Here's how the part is built. I have some questions about the finished solid (model axes, mm). A direction names the side the tool comes from. Round coordinates to 2 decimals unless told otherwise and drop trailing zeros. Loops run counter-clockwise (first coordinate to the right, second up) from the corner with the lowest first, then second, coordinate; pieces in that order, holes last. Notation, with made-up numbers: M 12,-30 L 32,-30 A30 cw 32,-7 Z; hole C 54.25,-12.5 d3. An arc over 180 degrees is marked long. Write each question's results on one line, items separated by ' | '. Start each with the question number.
Autodesk Fusion 360 part; units mm, degrees
sketch "Sketch1" plane through (0, 0, 0) normal (0, 0, 1) x (1, 0, 0)
  line L0 (3, 6) -> (38, 6)
  line L1 (38, 6) -> (38, -1)
  line L2 (38, -1) -> (3, -1)
  line L3 (3, -1) -> (3, 6)
  line L4 (3, 6) -> (5, 6)
  line L5 (5, 6) -> (5, -1)
  line L6 (5, -1) -> (3, -1)
  line L7 (3, -1) -> (3, 6)
  line L8 (5, 2.5) -> (12, 2.5)
  line L9 (12, 2.5) -> (12, 4)
  line L10 (12, 4) -> (5, 4)
  line L11 (5, 4) -> (5, 2.5)
  line L12 (5, 2.5) -> (12, 2.5)
  line L13 (12, 2.5) -> (12, 1)
  line L14 (12, 1) -> (5, 1)
  line L15 (5, 1) -> (5, 2.5)
  circle A0 centre (6.5, 2.5) radius 1.5
  circle A1 centre (10.5, 2.5) radius 1.5
  line L16 (3, -1) -> (13, -1)
  line L17 (13, -1) -> (13, 6)
  line L18 (13, 6) -> (3, 6)
  line L19 (3, 6) -> (3, -1)
  line L20 (13, 2.5) -> (20, 2.5)
  line L21 (20, 2.5) -> (20, 16)
  line L22 (20, 16) -> (13, 16)
  line L23 (13, 16) -> (13, 2.5)
  line L24 (13, 2.5) -> (20, 2.5)
  line L25 (20, 2.5) -> (20, -11)
  line L26 (20, -11) -> (13, -11)
  line L27 (13, -11) -> (13, 2.5)
  line L28 (20, 16) -> (20, 14)
  line L29 (13, 14) -> (13, 16)
  line L30 (13, -11) -> (20, -11)
  line L31 (20, -11) -> (20, -9)
  line L32 (13, -9) -> (13, -11)
  line L33 (20, -11) -> (20, -4)
  line L34 (20, -4) -> (13, -4)
  line L35 (13, -4) -> (13, -11)
  circle A2 centre (16.5, -7.5) radius 3.5
  circle A3 centre (16.5, -7.5) radius 1.5
  line L36 (13, 16) -> (20, 16)
  line L37 (20, 16) -> (20, 9)
  line L38 (20, 9) -> (13, 9)
  line L39 (13, 9) -> (13, 16)
  circle A4 centre (16.5, 12.5) radius 3.5
  circle A5 centre (16.5, 12.5) radius 1.5
  line L40 (38, 2.5) -> (23, 2.5)
  line L41 (23, 2.5) -> (23, 10)
  line L42 (23, 10) -> (38, 10)
  line L43 (38, 10) -> (38, 2.5)
  line L44 (23, 2.5) -> (38, 2.5)
  line L45 (38, 2.5) -> (38, -5)
  line L46 (38, -5) -> (23, -5)
  line L47 (23, -5) -> (23, 2.5)
  circle A6 centre (30.5, 2.5) radius 7.5
  circle A7 centre (30.5, 2.5) radius 1.5
  circle A8 centre (22.5, -3.5) radius 2.5
  circle A9 centre (22.5, 8.5) radius 2.5
  circle A10 centre (6.5, 2.5) radius 3.5
  circle A11 centre (10.5, 8.5) radius 2.5
  circle A12 centre (10.5, -3.5) radius 2.5
  dimension "d1" = 35
  dimension "d2" = 7
  dimension "d3" = 2
  dimension "d4" = 7
  dimension "d5" = 1.5
  dimension "d6" = 3
  dimension "d7" = 3
  dimension "d10" = 10
  dimension "d11" = 7
  dimension "d12" = 13.5
  dimension "d13" = 13.5
  dimension "d17" = 7
  dimension "d18" = 3
  dimension "d19" = 7
  dimension "d20" = 3
  dimension "d21" = 15
  dimension "d22" = 7.5
  dimension "d23" = 7.5
  dimension "d24" = 15
  dimension "d25" = 3
  dimension "d26" = 5
  dimension "d27" = 5
  dimension "d30" = 7
  dimension "d31" = 5
  dimension "d32" = 5
extrude "Extrude1" add sketch "Sketch1" along normal blind 2 contours L0 L3 L4 L5 L7 L18 L19 A10 | L0 L5 L18 A10 | L2 L3 L5 L6 L7 L16 L19 A10 | L5 L11 L15 A10 | L0 L2 L9 L10 L13 L14 L16 L17 L18 L23 L27 A10 | L5 L10 A10 | L2 L5 L16 A10 | L5 L14 A10 | L5 L10 L11 A0 | L5 L14 L15 A0 | L0 L21 L23 L38 | L0 L17 L20 L21 L23 L24 | L9 L10 A1 | L0 L21 A9 | L0 L2 L21 L25 L41 L47 | L2 L17 L20 L24 L25 L27 | L23 L38 L39 A4 | L13 L14 A1 | L2 L25 L27 L34 | A4 | L21 L37 L38 A4 | L2 L25 A8 | L27 L34 L35 A2 | L0 L41 A6 | A2 | L25 L33 L34 A2 | L0 A6 | L0 L40 L44 A6 A7 | L2 L47 A6 | L2 L40 L44 A6 A7 | L2 A6
extrude "Extrude2" add sketch "Sketch1" along normal blind 2 contours L2 L16 L27 A12
extrude "Extrude3" add sketch "Sketch1" along normal blind 2 contours L0 L18 L23 A11
extrude "Extrude4" cut sketch "Sketch1" along normal blind 2 contours L0 L3 L4 L5 L7 L18 L19 A10
extrude "Extrude5" cut sketch "Sketch1" along normal blind 2 contours L0 L5 L18 A10 | L2 L3 L5 L6 L7 L16 L19 A10 | L2 L5 L16 A10
Item 1: If we mould it in two halves opening along Y, with no side actions, what happens to faces 4 (the face through (9, 4, 1)), 5 (the face through (37.995, 2.779, 0.986)), 6 (the face through (20, 10, 1)), 7 (the face through (15, 12.43, 0.99))? For each: released by +Y, released by -Y, zero draft, split by the parting line, or undercut.
Item 2: If we section it at C-C on y = -1.75: Please give me the cut outline in (x, z).
Item 3: If we section it at A-A on x = 16.5: Please give me the cut outline in (y, z), and give its area (3 significant figures).
Item 4: I need wall thicknesses on L1, parallel to Y at x = 16.5, z = 0.55; L2, parallel to X at y = 2.5, z = 1.1; L3, parallel to X at y = 3.75, z = 0.45. Which ranges of each line are inside material? Lowest first, please.
Item 5: If we section it at B-B on z = 1.5: Please give me the cut outline in (x, y), and give its area (3 significant figures).
Item 6: Which directions (+Z, -Z, +X, -X, +Y, -Y) give clear straight access to the entire face, cutting with the end or side of a thin tool? Please do faces 1 (the face through (13, 11, 1)), 2 (the face through (20, -5, 1)), 3 (the face through (20.752, 6.713, 0.986)).
Item 7: If we section it at D-D on x = 8: Please give me the cut outline in (y, z), and give its area (3 significant figures).
Item 8: I'm going to push flat-ended pins straight in: pin 1 (0.6 mm diameter, centred on x = 8, z = 1.5, fed in from -Y); pin 2 (1.8 mm diameter, centred on x = 30.5, y = 2.5, fed in from -Z); pin 3 (0.6 mm diameter, centred on y = -6, z = 0.5, fed in from -X). Where does each tip first touch, or does it pass through?
Numbers:
1) face 4: undercut | face 5: split by the parting line | face 6: zero draft | face 7: undercut
2) outline: M 12.29,0 L 20.71,0 L 20.71,2 L 12.29,2 Z; M 24.32,0 L 36.68,0 L 36.68,2 L 24.32,2 Z
3) outline: M -11,0 L -9,0 L -9,2 L -11,2 Z; M -6,0 L 11,0 L 11,2 L -6,2 Z; M 14,0 L 16,0 L 16,2 L 14,2 Z | area: 42.0 mm²
4) L1: -11 to -9, -6 to 11, 14 to 16 | L2: 3 to 5, 12 to 29, 32 to 38 | L3: 3.23 to 5.67, 11.33 to 29.67, 31.33 to 37.9
5) outline: M 6.5,-1 L 10.5,-1 A2.5 cw 13,-3.5 L 13,-7.5 A3.5 ccw 20,-7.5 L 20,-3.5 A2.5 cw 22.5,-1 L 23.87,-1 A7.5 ccw long 23.87,6 L 22.5,6 A2.5 cw 20,8.5 L 20,12.5 A3.5 ccw 13,12.5 L 13,8.5 A2.5 cw 10.5,6 L 6.5,6 A3.5 ccw Z; hole M 6.5,1 L 10.5,1 A1.5 ccw 10.5,4 L 6.5,4 A1.5 ccw Z; hole C 16.5,-7.5 d3; hole C 16.5,12.5 d3; hole C 30.5,2.5 d3 | area: 408 mm²
6) face 1: +Z, -Z, -X, +Y | face 2: +Z, -Z, -Y | face 3: +Z, -Z, +Y
7) outline: M -1,0 L 1,0 L 1,2 L -1,2 Z; M 4,0 L 6,0 L 6,2 L 4,2 Z | area: 8.00 mm²
8) pin 1: y = -1 | pin 2: through | pin 3: x = 13
